Autodesk Inventor part; units mm, degrees
ref_plane "Start plane" through (0, 0, -21.042) normal (0, 0, 1) x (1, 0, 0)
ref_plane "End plane" through (0, 0, 353.3115) normal (0, 0, 1) x (1, 0, 0)
ref_plane "Work Plane3" through (50.8, 38.1, -21.042) normal (-0.3827, 0, -0.9239) x (-0.9239, 0, 0.3827)
ref_plane "Start plane" through (0, 0, -21.042) normal (0, 0, 1) x (1, 0, 0)
ref_plane "End plane" through (0, 0, 353.3115) normal (0, 0, 1) x (1, 0, 0)
sketch "Sketch" plane through (0, 0, 0) normal (0, 0, 1) x (1, 0, 0)
  line L0 (0, 76.2) -> (0, 0)
  line L1 (0, 0) -> (50.8, 0)
  line L2 (50.8, 0) -> (50.8, 2.7625)
  line L3 (48.8, 4.7625) -> (12.6365, 4.7625)
  line L4 (4.7625, 12.6365) -> (4.7625, 74.2)
  line L5 (2.7625, 76.2) -> (0, 76.2)
  line L6 (-7.0414, 0) -> (21.5385, 0) construction
  line L7 (0, -8.0414) -> (0, 34.5385) construction
  arc A0 (4.7625, 12.6365) -> (12.6365, 4.7625) centre (12.6365, 12.6365) ccw
  arc A1 (50.8, 2.7625) -> (48.8, 4.7625) centre (48.8, 2.7625) ccw
  arc A2 (4.7625, 74.2) -> (2.7625, 76.2) centre (2.7625, 74.2) ccw
  line L8 (0, 93.5453) -> (0, -24.9725) construction
  line L9 (-18.6925, 0) -> (62.8653, 0) construction
  point P0 (50.8, 4.7625)
  point P1 (4.7625, 4.7625)
  point P2 (4.7625, 76.2)
  dimension "d12" = 4.7625
  dimension "d13" = 76.2
  dimension "d14" = 50.8
  dimension "d15" = 0
  dimension "d16" = 4.7625
  dimension "d17" = 0
  dimension "d18" = 7.874
  dimension "d19" = 2
extrude "Body" add sketch "Sketch" along normal up to surface (374.3536 mm away) from surface at -21.042
ref_plane "Work Plane3" through (50.8, 38.1, -21.042) normal (-0.3827, 0, -0.9239) x (-0.9239, 0, 0.3827)
split "Split1" plane through (50.8, 38.1, -21.042) removes the side toward (-0.3827, 0, -0.9239)
ref_plane "Work Plane4" through (50.8, 38.1, 353.3115) normal (-0.3827, 0, 0.9239) x (0.9239, 0, 0.3827)
split "Split2" plane through (50.8, 38.1, 353.3115) removes the side toward (-0.3827, 0, 0.9239)
equation "\"d12\" = G_T"
equation "\"d13\" = G_H"
equation "\"d14\" = G_W"
equation "\"d16\" = G_T"
equation "\"d18\" = G_IR"
equation "\"d4\" = G_L"
equation "\"G_W\" = 50.8"
equation "\"G_H\" = 76.2"
equation "\"G_T\" = 4.7625"
equation "\"G_ER\" = 4.064"
equation "\"G_IR\" = 7.874"
equation "\"G_L\" = B_L + G_OFFSET_START + G_OFFSET_END"
equation "\"ex\" = 0"
equation "\"ey\" = 0"
equation "\"G_OFFSET_START\" = 21.04205"
equation "\"G_OFFSET_END\" = 21.04205"
equation "\"d20\" = -G_OFFSET_START"
equation "\"d21\" = G_OFFSET_END + B_L"
equation "\"B_L\" = 332.26948"
properties part number "ANSI L 3 x 2 x 3_16 00000012"
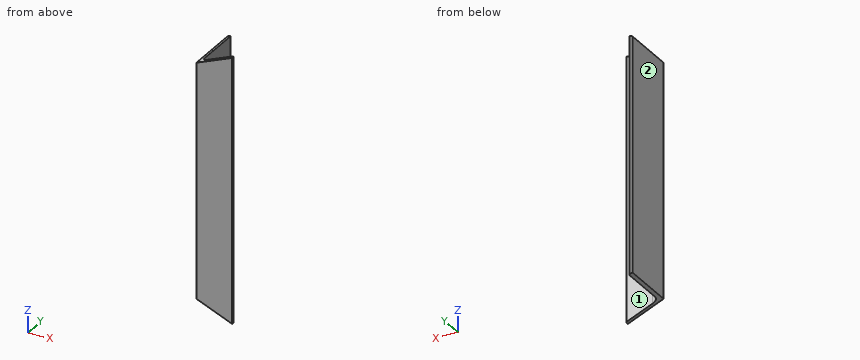
The listing builds one solid part. Answer for the finished solid, in the listing's coordinates (mm). Face numbers are marked on the shaded views. A direction names the side the tool comes from. Give positions to 0.01 mm unless a question says otherwise; leave off trailing zeros. Write each loop counter-clockwise with the first axis right and the second up, starting at its lowest first coordinate (ties: lowest second). Pieces come first, ordered by that corner, then holes. Notation, with made-up numbers: M 87,-29 L 139,-29 A24 ccw 139,-18 Z; hole C -28.75,17 d10. An arc over 180 degrees is marked long. Write each question's results on one line, items separated by ' | '.
Q1. A tool of negligible diameter and unlimited length cuts with its end or side. For the marked faces 1 and 2, from which of +Z, -Z, +X, -X, +Y, -Y can it reach the whole face along a straight path? Write none if from no direction.
Output values:
face 1: +Z, -Z, +X, +Y | face 2: +Z, -Z, -X, +Y, -Y
Q2. Flat-ended cylindrical pins translate along their axes: P1, Ø18.5, axis at y = 46.5, z = 89.5, coming from the +X side; P2, Ø11, axis at x = 28, z = 258.5, coming from the +Y side. Find the tip coordinate at first contact, or state that the pin passes through.
Output values:
P1: x = 4.76 | P2: y = 4.76
Q3. Section B-B, the plane y = 61.5 is taken. Write down the section's boundary in (x, z), then the cut area to 3 significant figures.
Output values:
outline: M 0,0 L 4.76,-1.97 L 4.76,334.24 L 0,332.27 Z | area: 1,590 mm2
Q4. Consider L1, parallel to X at y = 32, z = 297.5; L2, parallel to Y at x = 5.5, z = 19. Determine where each line is inside the solid, lowest interval first. Write a range as from..to.
Output values:
L1: 0..4.76 | L2: 0..9.31
Q5. Section A-A, the plane z = 152 is taken. Write down the section's boundary in (x, y), then the cut area to 3 significant figures.
Output values:
outline: M 0,0 L 50.8,0 L 50.8,2.76 A2 ccw 48.8,4.76 L 12.64,4.76 A7.87 cw 4.76,12.64 L 4.76,74.2 A2 ccw 2.76,76.2 L 0,76.2 Z | area: 594 mm2
Q6. Section C-C, the plane x = 21.5 is taken. Write down the section's boundary in (y, z), then the cut area to 3 significant figures.
Output values:
outline: M 0,-8.91 L 4.76,-8.91 L 4.76,341.18 L 0,341.18 Z | area: 1,670 mm2
